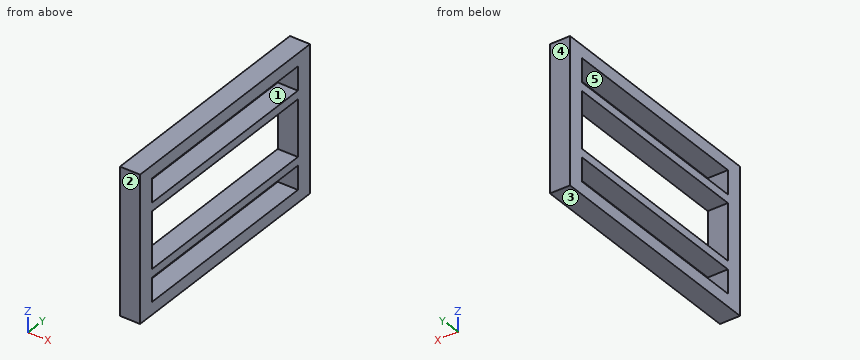
```python
from build123d import *

# Parameters (mm, degrees)
SKETCH1_W           = 4.8
SKETCH1_H           = 34.8
BOSS_EXTRUDE1_DEPTH = 56
SKETCH2_W           = 5.67
SKETCH2_H           = 48
SKETCH2_W_2         = 13.46
CUT_EXTRUDE1_DEPTH  = 56


with BuildPart() as part:
    # Sketch1 → Boss-Extrude1 (new body)
    with BuildSketch(Plane(origin=(0, 0, 0), x_dir=(1, 0, 0), z_dir=(0, 1, 0))):
        with Locations((-0.073796791, 12.667379679)):
            Rectangle(SKETCH1_W, SKETCH1_H)
    extrude(amount=BOSS_EXTRUDE1_DEPTH)

    # Sketch2 → Cut-Extrude1 (cut)
    with BuildSketch(Plane(origin=(2.326203209, 0, 0), x_dir=(0, 0, -1), z_dir=(1, 0, 0))):
        with Locations((1.102379679, 28)):
            Rectangle(SKETCH2_W, SKETCH2_H)
        with Locations((12.667379679, 28)):
            Rectangle(SKETCH2_W_2, SKETCH2_H)
        with Locations((24.232379679, 28)):
            Rectangle(SKETCH2_W, SKETCH2_H)
    extrude(amount=-CUT_EXTRUDE1_DEPTH, mode=Mode.SUBTRACT)


solid = part.part
```
Input: part model. Units: mm. Frame: model coordinates. Face numbers are marked on the shaded views. A direction names the side the tool comes from. Coordinates: 2 decimals unless noted, no trailing zeros. Write each loop counter-clockwise with the first axis right and the second up, starting at its lowest first coordinate (ties: lowest second). Pieces come first, ordered by that corner, then holes. Notation, with made-up numbers: (80, 73.5) -> (94, 73.5) arc R23 ccw to (94, 97.5) -> close; hole circle Ø3 at (9.5, -31.5). An arc over 180 degrees is marked (long way). Answer as a JSON object with one key per item and string values.
1. Section B-B on y = 19.5. Return the cut outline in (x, z), then the cut area to 3 significant figures.
Result set:
{"outline": "(-2.47, -30.07) -> (2.33, -30.07) -> (2.33, -27.07) -> (-2.47, -27.07) -> close; (-2.47, -21.4) -> (2.33, -21.4) -> (2.33, -19.4) -> (-2.47, -19.4) -> close; (-2.47, -5.94) -> (2.33, -5.94) -> (2.33, -3.94) -> (-2.47, -3.94) -> close; (-2.47, 1.73) -> (2.33, 1.73) -> (2.33, 4.73) -> (-2.47, 4.73) -> close", "area": "48.0 mm2"}
2. Material intervals for line 1 (Z direction, x = -1.6, y = 16); line 2 (Y direction, x = 1.15, z = -9), sorted ascending. Write a range as from..to.
Result set:
{"line 1": "z = -30.07..-27.07, -21.4..-19.4, -5.94..-3.94, 1.73..4.73", "line 2": "y = 0..4, 52..56"}
3. Mould query, pull axis Z, two halves, no side actions, for the marked faces 1, 2 and 3. Classes: released by +Z, released by -Z, zero draft, split by the parting line, or undercut.
Result set:
{"face 1": "undercut", "face 2": "zero draft", "face 3": "released by -Z"}
4. Section A-A on z = -11. Return the cut outline in (x, y).
Result set:
{"outline": "(-2.47, 0) -> (2.33, 0) -> (2.33, 4) -> (-2.47, 4) -> close; (-2.47, 52) -> (2.33, 52) -> (2.33, 56) -> (-2.47, 56) -> close"}
5. Section C-C on x = -0.45. Return the cut outline in (y, z), then the cut area to 3 significant figures.
Result set:
{"outline": "(0, -30.07) -> (56, -30.07) -> (56, 4.73) -> (0, 4.73) -> close; hole (4, -27.07) -> (52, -27.07) -> (52, -21.4) -> (4, -21.4) -> close; hole (4, -19.4) -> (52, -19.4) -> (52, -5.94) -> (4, -5.94) -> close; hole (4, -3.94) -> (52, -3.94) -> (52, 1.73) -> (4, 1.73) -> close", "area": "758 mm2"}
6. Access query for the marked faces 4 and 5. Directions: +Z, -Z, +X, -X, +Y, -Y. A direction counts if a zero-diameter tool reaches every point of the face in a straight line with its end or side. Return the directions, or none.
Result set:
{"face 4": "+Z, -Z, +X, -X, +Y", "face 5": "+X, -X"}
